```python
from build123d import *

# Parameters (mm, degrees)
SKETCH1_R           = 14.2875
SKETCH1_R_2         = 2.54
BOSS_EXTRUDE1_DEPTH = 3.175
CUT_EXTRUDE1_DEPTH  = 162.674043733
FILLET3_R           = 6.35
SKETCH3_R           = 2.54
BOSS_EXTRUDE3_DEPTH = 3.175
SKETCH6_R           = 2.54
BOSS_EXTRUDE4_DEPTH = 3.175
FILLET2_R           = 6.35
CUT_EXTRUDE2_DEPTH  = 169.237022961
CUT_EXTRUDE3_DEPTH  = 169.237022961
CUT_EXTRUDE4_DEPTH  = 168.265702461
BOSS_EXTRUDE7_DEPTH = 3.175
SKETCH14_R          = 14.2875
BOSS_EXTRUDE8_DEPTH = 3.175
SKETCH15_R          = 14.2875
CUT_EXTRUDE5_DEPTH  = 128.70732581
CUT_EXTRUDE6_DEPTH  = 128.70732581
SKETCH17_R          = 2.54
CUT_EXTRUDE7_DEPTH  = 128.70732581


with BuildPart() as part:
    # Sketch1 → Boss-Extrude1 (new body)
    with BuildSketch(Plane.XY):
        with BuildLine():
            Line((-8.89, 25.4), (8.89, 25.4))
            ThreePointArc((8.89, 25.4), (17.870256121, 21.680256121), (21.59, 12.7))
            Line((21.59, 12.7), (21.59, -117.775079775))
            ThreePointArc((21.59, -117.775079775), (21.127743647, -120.388718212), (19.797058824, -122.685251408))
            Line((19.797058824, -122.685251408), (-7.952696208, -155.616779465))
            ThreePointArc((-7.952696208, -155.616779465), (-12.268297602, -157.851943494), (-16.900388255, -156.380852124))
            Line((-16.900388255, -156.380852124), (-32.439211784, -143.287061102))
            ThreePointArc((-32.439211784, -143.287061102), (-34.674375812, -138.971459708), (-33.203284443, -134.339369055))
            Line((-33.203284443, -134.339369055), (-23.382941176, -122.685251408))
            ThreePointArc((-23.382941176, -122.685251408), (-22.052256353, -120.388718212), (-21.59, -117.775079775))
            Line((-21.59, -117.775079775), (-21.59, 12.7))
            ThreePointArc((-21.59, 12.7), (-17.870256121, 21.680256121), (-8.89, 25.4))
        make_face()
        Circle(SKETCH1_R, mode=Mode.SUBTRACT)
        with Locations((0, -101.6)):
            Circle(SKETCH1_R, mode=Mode.SUBTRACT)
        with Locations((-18.532085478, -142.550133084)):
            Circle(SKETCH1_R_2, mode=Mode.SUBTRACT)
        with Locations((0, -50.8)):
            Circle(SKETCH1_R_2, mode=Mode.SUBTRACT)
    extrude(amount=BOSS_EXTRUDE1_DEPTH)

    # Sketch2 → Cut-Extrude1 (cut, through all)
    with BuildSketch(Plane.XY):
        with BuildLine():
            ThreePointArc((19.159083004, -91.647229609), (9.182340769, -50.8), (19.159083004, -9.952770391))
            ThreePointArc((19.159083004, -9.952770391), (20.973467787, -5.122670102), (21.59, 0))
            Line((21.59, 0), (27.94, 0))
            Line((27.94, 0), (27.94, -121.656687185))
            Line((27.94, -121.656687185), (-7.620284479, -163.8572221))
            Line((-7.620284479, -163.8572221), (-17.501317584, -155.874478972))
            Line((-17.501317584, -155.874478972), (16.51, -115.512152961))
            ThreePointArc((16.51, -115.512152961), (20.280273667, -109.005308906), (21.59, -101.6))
            ThreePointArc((21.59, -101.6), (20.973467787, -96.477329898), (19.159083004, -91.647229609))
        make_face()
        with BuildLine():
            Line((-21.59, -41.275), (-21.59, -60.325))
            ThreePointArc((-21.59, -60.325), (-12.065, -50.8), (-21.59, -41.275))
        make_face()
    extrude(amount=CUT_EXTRUDE1_DEPTH, mode=Mode.SUBTRACT)


with BuildPart() as cut_extrude1_piece_1:
    # of the separate pieces the step leaves, piece 1, a body of its own (cut_extrude1_pieces)
    add(part.part.solids().sort_by_distance((-8.89, 25.4, 0))[0])

    # Fillet3
    fillet3_edges = [cut_extrude1_piece_1.edges().sort_by_distance(p)[0] for p in [
        (-21.59, -41.275, 1.5875),
        (-21.59, -60.325, 1.5875),
    ]]
    fillet(fillet3_edges, radius=FILLET3_R)

    # Sketch3 → Boss-Extrude3 (add)
    with BuildSketch(Plane.XY.offset(3.175)):
        with BuildLine():
            Line((-27.351416194, -127.394768527), (-36.025496499, -137.688579))
            ThreePointArc((-36.025496499, -137.688579), (-37.217489152, -141.441859142), (-35.4063854, -144.93869507))
            Line((-35.4063854, -144.93869507), (-24.403104784, -154.210610454))
            ThreePointArc((-24.403104784, -154.210610454), (-19.771014132, -155.681701823), (-15.455412737, -153.446537795))
            Line((-15.455412737, -153.446537795), (-7.557639641, -144.073996091))
            Line((-7.557639641, -144.073996091), (-27.351416194, -127.394768527))
        make_face()
        with Locations((-18.532085478, -142.550133084)):
            Circle(SKETCH3_R, mode=Mode.SUBTRACT)
    extrude(amount=-BOSS_EXTRUDE3_DEPTH)

    # Sketch6 → Boss-Extrude4 (add)
    with BuildSketch(Plane.XY.offset(3.175)):
        Polygon((-35.4063854, -144.93869507), (-63.620410749, -121.164144113), (-51.344981666, -106.596497054), (-27.065569901, -127.055545526), align=None)
        with Locations((-52.626813855, -117.972130278)):
            Circle(SKETCH6_R, mode=Mode.SUBTRACT)
    extrude(amount=-BOSS_EXTRUDE4_DEPTH)

    # Fillet2
    fillet2_edges = [cut_extrude1_piece_1.edges().sort_by_distance(p)[0] for p in [
        (-63.620410749, -121.164144113, 1.5875),
        (-51.344981666, -106.596497054, 1.5875),
        (-27.065569901, -127.055545526, 1.5875),
    ]]
    fillet(fillet2_edges, radius=FILLET2_R)

    # Sketch7 → Cut-Extrude2 (cut, through all)
    with BuildSketch(Plane.XY.offset(3.175)):
        with BuildLine():
            Line((-21.59, 0), (-21.59, 31.75))
            Line((-21.59, 31.75), (21.59, 31.75))
            Line((21.59, 31.75), (21.59, 0))
            ThreePointArc((21.59, 0), (0, 21.59), (-21.59, 0))
        make_face()
    extrude(amount=-CUT_EXTRUDE2_DEPTH, mode=Mode.SUBTRACT)


with BuildPart() as cut_extrude1_piece_2:
    # of the separate pieces the step leaves, piece 2, a body of its own (cut_extrude1_pieces)
    add(part.part.solids().sort_by_distance((-16.900388255, -156.380852124, 0))[0])


with BuildPart() as cut_extrude3_tool:
    # Sketch10 → Cut-Extrude3 (new, through all)
    with BuildSketch(Plane.XY.offset(3.175)):
        with BuildLine():
            Line((-18.151882461, -155.32628042), (-17.361482582, -157.512020269))
            Line((-17.361482582, -157.512020269), (-14.375706423, -156.432313955))
            Line((-14.375706423, -156.432313955), (-15.455412737, -153.446537795))
            ThreePointArc((-15.455412737, -153.446537795), (-16.679911193, -154.563907595), (-18.151882461, -155.32628042))
        make_face()
    extrude(amount=-CUT_EXTRUDE3_DEPTH)


with BuildPart() as cut_extrude1_piece_1_1:
    add(cut_extrude1_piece_1.part)

    # Cut-Extrude3: cut by cut_extrude3_tool
    add(cut_extrude3_tool.part, mode=Mode.SUBTRACT)

    # Sketch12 → Cut-Extrude4 (cut, through all)
    with BuildSketch(Plane.XY.offset(3.175)):
        with BuildLine():
            Line((-21.59, -101.6), (-72.39, -101.6))
            Line((-72.39, -101.6), (-72.39, -165.1))
            Line((-72.39, -165.1), (16.51, -165.1))
            Line((16.51, -165.1), (16.51, -115.512152961))
            ThreePointArc((16.51, -115.512152961), (-7.405308906, -121.880273667), (-21.59, -101.6))
        make_face()
    extrude(amount=-CUT_EXTRUDE4_DEPTH, mode=Mode.SUBTRACT)

    # Sketch13 → Boss-Extrude7 (add, through all)
    with BuildSketch(Plane.XY.offset(3.175)):
        with BuildLine():
            Line((-21.59, -101.6), (-21.59, -104.23906))
            ThreePointArc((-21.59, -104.23906), (0, -125.82906), (21.59, -104.23906))
            Line((21.59, -104.23906), (21.59, -101.6))
            Line((21.59, -101.6), (6.662926134, -118.366401535))
            Line((6.662926134, -118.366401535), (-7.350026675, -118.366401535))
            Line((-7.350026675, -118.366401535), (-21.59, -101.6))
        make_face()
    extrude(amount=-BOSS_EXTRUDE7_DEPTH)

    # Sketch14 → Boss-Extrude8 (add, through all)
    with BuildSketch(Plane.XY.offset(3.175)):
        with Locations((0, -101.6)):
            Circle(SKETCH14_R)
    extrude(amount=-BOSS_EXTRUDE8_DEPTH)

    # Sketch15 → Cut-Extrude5 (cut, through all)
    with BuildSketch(Plane.XY.offset(3.175)):
        with Locations((0, -104.23906)):
            Circle(SKETCH15_R)
    extrude(amount=-CUT_EXTRUDE5_DEPTH, mode=Mode.SUBTRACT)

    # Sketch16 → Cut-Extrude6 (cut, through all)
    with BuildSketch(Plane.XY.offset(3.175)):
        with BuildLine():
            Line((19.159083004, -91.647229609), (21.59, -91.647229609))
            Line((21.59, -91.647229609), (21.59, -104.23906))
            ThreePointArc((21.59, -104.23906), (20.97671132, -97.826892854), (19.159083004, -91.647229609))
        make_face()
    extrude(amount=-CUT_EXTRUDE6_DEPTH, mode=Mode.SUBTRACT)

    # Sketch17 → Cut-Extrude7 (cut, through all)
    with BuildSketch(Plane(origin=(0, 0, 0), x_dir=(-1, 0, 0), z_dir=(0, 0, -1))):
        with Locations((12.7, -19.05)):
            Circle(SKETCH17_R)
        with Locations((12.7, -82.55)):
            Circle(SKETCH17_R)
        with Locations(Location((0, -50.8, 0), (0, 0, 180))):
            Circle(SKETCH17_R)
    extrude(amount=-CUT_EXTRUDE7_DEPTH, mode=Mode.SUBTRACT)


with BuildPart() as cut_extrude1_piece_2_1:
    add(cut_extrude1_piece_2.part)

    # Cut-Extrude3: cut by cut_extrude3_tool
    add(cut_extrude3_tool.part, mode=Mode.SUBTRACT)


solid = cut_extrude1_piece_1_1.part
```
Build history of the part. All positions in model axes, mm. A direction names the side the tool comes from. Give positions to 0.01 mm unless a question says otherwise; leave off trailing zeros. Loops run counter-clockwise (first coordinate to the right, second up) from the corner with the lowest first, then second, coordinate; pieces in that order, holes last. Notation, with made-up numbers: (-18, 3.25) - (31, 3.25) arc R17 cw to (31, 36.25) - close; hole circle Ø6 at (13, -39.75). An arc over 180 degrees is marked (long way). Use a Markdown table: item, result.
(1) Pull direction Y, two halves, no side cores. Call faces 4 (the face through (-5, -51, 3.175)), 5 (the face through (-0.475, -125.824, 1.61)), 6 (the face through (-12.37, -16.53, 1.57)): +Y half, -Y half, draft (parallel to the pull), parting line (faces both ways), or undercut.
Taken from the geometry:
| item | result |
|---|---|
| face 4 | draft |
| face 5 | -Y half |
| face 6 | undercut |
(2) Band-saw the part on D-D (y = -82.55). Give the cut face in (x, z) (3 decimals), and give its area (3 significant figures).
Taken from the geometry:
| item | result |
|---|---|
| outline | (-21.59, 0) - (-15.24, 0) - (-15.24, 3.175) - (-21.59, 3.175) - close; (-10.16, 0) - (15.066, 0) - (15.066, 3.175) - (-10.16, 3.175) - close |
| area | 100 mm2 |
(3) Drop a flat-ended pin along its axis: pin 1 Ø1.5 at (x, z) = (-2.5, 1) entering from -Y. Give the stop position or say it passes through.
Taken from the geometry:
| item | result |
|---|---|
| pin 1 | y = -125.76 |
(4) Band-saw the part on B-B (x = 0). Give the cut face in (y, z) (1 decimal).
Taken from the geometry:
| item | result |
|---|---|
| outline | (-125.8, 0) - (-118.5, 0) - (-118.5, 3.2) - (-125.8, 3.2) - close; (-90, 0) - (-53.3, 0) - (-53.3, 3.2) - (-90, 3.2) - close; (-48.3, 0) - (-14.3, 0) - (-14.3, 3.2) - (-48.3, 3.2) - close; (14.3, 0) - (21.6, 0) - (21.6, 3.2) - (14.3, 3.2) - close |
(5) Band-saw the part on A-A (z = 1.3). Give the number of separate pieces and of enclosed holes in the cut face, and give its area (3 significant figures).
Taken from the geometry:
| item | result |
|---|---|
| separate pieces | 1 |
| enclosed holes | 5 |
| area | 3,700 mm2 |
(6) Band-saw the part on C-C (y = -50.8). Give the cut face in (x, z) (3 decimals).
Taken from the geometry:
| item | result |
|---|---|
| outline | (-12.065, 0) - (-2.54, 0) - (-2.54, 3.175) - (-12.065, 3.175) - close; (2.54, 0) - (9.182, 0) - (9.182, 3.175) - (2.54, 3.175) - close |
(7) Which spindle directions (+Z, -Z, +X, -X, +Y, -Y) get a long thin tool onto all of the face, cutting with end or side? Do faces 1 (the face through (20.994, -97.916, 1.61)), 2 (the face through (-3.097, -118.187, 1.61)), 3 (the face through (-20.524, -61.829, 1.61)). Say none if no direction does.
Taken from the geometry:
| item | result |
|---|---|
| face 1 | +Z, -Z, +X |
| face 2 | +Z, -Z |
| face 3 | +Z, -Z, -X |
(8) Wall check: line 1 along Y through (x, z) = (0, 1.75); line 2 along Y through (x, z) = (-12, 1.85); line 3 along Y through (x, z) = (-5.5, 1.1). Give the ranges that are in metal, low to high.
Taken from the geometry:
| item | result |
|---|---|
| line 1 | -125.83 to -118.53, -89.95 to -53.34, -48.26 to -14.29, 14.29 to 21.59 |
| line 2 | -122.19 to -111.99, -96.48 to -84.99, -80.11 to -21.49, -16.61 to -7.75, 7.75 to 17.95 |
| line 3 | -125.12 to -117.43, -91.05 to -13.19, 13.19 to 20.88 |
